Check sheet for the drawn part. Datum: minimum x, y, z corner. Units: mm. A direction names the side the tool comes from. Give positions to 0.01 mm unless a question says otherwise; leave off trailing zeros. Order: outer loops, then holes, each group sorted by start corner. A loop starts at its lowest first (then second) coordinate and runs counter-clockwise, first axis right, second up. Notation, with made-up numbers: (55, 3) - (68, 3) arc R11 cw to (68, 15) - close; hole circle Ø1 at (78, 71). An arc over 180 degrees is marked (long way). Answer as a JSON object with one key per item and string values. Group by question number.
(1) Thickness scan on line 1 (X direction, y = 1.25, z = 5); line 2 (X direction, y = 3.75, z = 6.5); line 3 (Y direction, x = 16, z = 5). Record the ranges inside material, lowest first.
(2) Access from +Z, -Z, +X, -X, +Y, -Y to the whole of each face (thin tool, end or side, straight path). Record for the marked faces 1 and 2.
(3) Section check A-A (z = 5). Record the boundary of the cut face in (x, y).
(4) Mould release check, pull along Y, two halves, no side actions. Record for the marked faces 3, 4 and 5: +Y half, -Y half, draft (parallel to the pull), parting line (faces both ways), or undercut.
(5) Section check B-B (x = 32). Record the boundary of the cut face in (y, z).
(6) Depth check by flat-ended pin: pin 1 Ø6 at (x, y) = (11.5, 8) entering from -Z; pin 2 Ø0.8 at (x, z) = (1, 5.5) entering from +Y; pin 3 Ø6 at (x, z) = (13.5, 1.5) entering from -Y; pin 4 Ø4 at (x, y) = (38, 5.5) entering from +Z. Enter the tip coordinate at first touch or a pass-through.
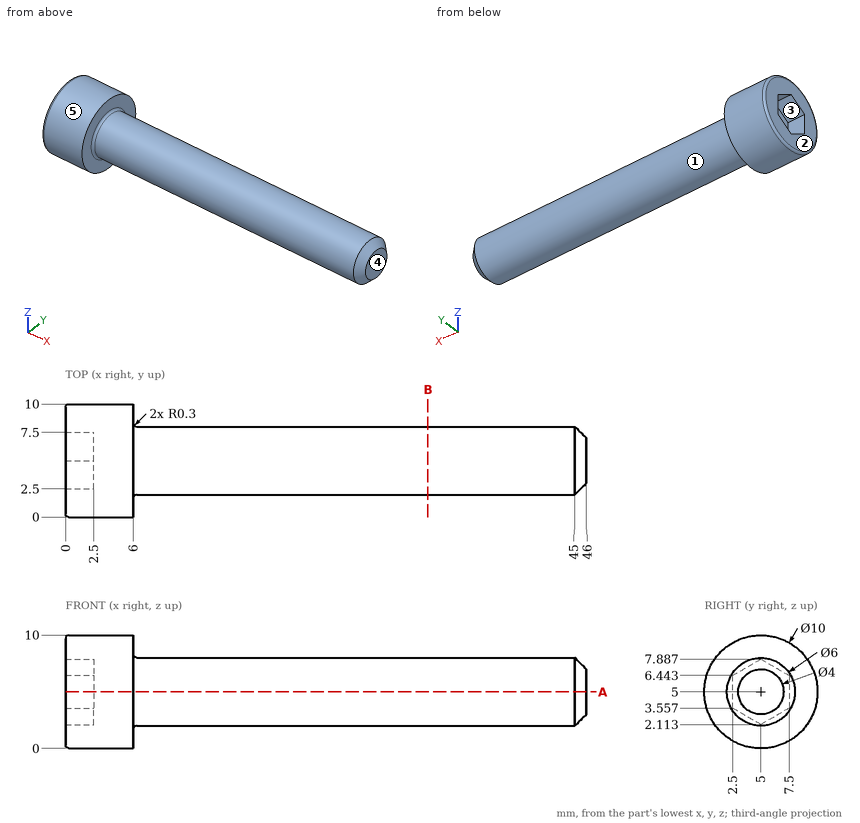
Solutions:
{
 "1": {"line 1": "x = 0 to 6", "line 2": "x = 2.5 to 46", "line 3": "y = 2 to 8"},
 "2": {"face 1": "+X", "face 2": "+Z, -Z, -X, +Y, -Y"},
 "3": {"outline": "(0, 0.3) arc R0.3 ccw to (0.3, 0) - (6, 0) - (6, 1.7) arc R0.3 cw to (6.3, 2) - (45, 2) - (46, 3) - (46, 7) - (45, 8) - (6.3, 8) arc R0.3 cw to (6, 8.3) - (6, 10) - (0.3, 10) arc R0.3 ccw to (0, 9.7) - (0, 7.5) - (2.5, 7.5) - (2.5, 2.5) - (0, 2.5) - close"},
 "4": {"face 3": "undercut", "face 4": "draft", "face 5": "parting line"},
 "5": {"outline": "circle Ø6 at (5, 5)"},
 "6": {"pin 1": "stops at z = 2", "pin 2": "stops at y = 10", "pin 3": "stops at y = 2.04", "pin 4": "stops at z = 8"}
}
